```python
from build123d import *

# Parameters (mm, degrees)
F0_W     = 157.873229
F0_H     = 63.821092
F1_DEPTH = 34
F3_DEPTH = 63.821092


with BuildPart() as f1:
    # F0 (on Front) → F1 (new body, symmetric)
    with BuildSketch(Plane.XZ):
        with Locations((19.16913, 67.018941)):
            Rectangle(F0_W, F0_H)
    extrude(amount=F1_DEPTH, both=True)

    # F2 (on face) → F3 (intersect, through all)
    with BuildSketch(Plane.XY.offset(98.929487)):
        with BuildLine():
            Line((-59.767485, 34), (-59.767485, -34))
            Line((-59.767485, -34), (88.105744, -34))
            ThreePointArc((88.105744, -34), (95.553897, -17.720045), (98.105744, 0))
            ThreePointArc((98.105744, 0), (95.553897, 17.720045), (88.105744, 34))
            Line((88.105744, 34), (-59.767485, 34))
        make_face()
    extrude(amount=-F3_DEPTH, mode=Mode.INTERSECT)


solid = f1.part
```
Here's how the part is built. I have some questions about the finished solid (model axes, mm). Round coordinates to 2 decimals unless told otherwise and drop trailing zeros. Loops run counter-clockwise (first coordinate to the right, second up) from the corner with the lowest first, then second, coordinate; pieces in that order, holes last.
1. Suppose I cut it at B-B, the plane y = -23. Please give me the cut outline in (x, z).
Answers:
outline: (-59.77, 35.11) - (93.74, 35.11) - (93.74, 98.93) - (-59.77, 98.93) - close
2. If I drill on probe 1 along Y at (x, z) = (90, 90); probe 2 along X at (y, z) = (-11, 51); probe 3 along X at (y, z) = (-12, 45), over which ranges is the centre line in solid material (lowest first)?
Answers:
probe 1: y = -30.86 to 30.86
probe 2: x = -59.77 to 97.13
probe 3: x = -59.77 to 96.95
3. Will these pins go through, and if not, where does the flat tip stop? pin 1 (5 mm diameter, centred on y = 23, z = 58, fed in from +X); pin 2 (2 mm diameter, centred on y = -14, z = 55, fed in from +X).
Answers:
pin 1: stops at x = 94.67
pin 2: stops at x = 96.75
4. Suppose I cut it at A-A, the plane z = 64.5. Please give me the cut outline in (x, y).
Answers:
outline: (-59.77, -34) - (88.11, -34) arc R62.8 ccw to (98.11, 0) arc R62.8 ccw to (88.11, 34) - (-59.77, 34) - close
5. Suppose I cut it at C-C, the plane y = 18. Please give me the cut outline in (x, z).
Answers:
outline: (-59.77, 35.11) - (95.47, 35.11) - (95.47, 98.93) - (-59.77, 98.93) - close
